Verification items for the finished model (mm, model axes). A direction names the side the tool comes from. Coordinates: 2 decimals unless noted, no trailing zeros. Order: outer loops, then holes, each group sorted by start corner. A loop starts at its lowest first (then second) coordinate and runs counter-clockwise, first axis right, second up. Notation, with made-up numbers: (20, 8) -> (58, 8) arc R25 ccw to (58, 28) -> close; hole circle Ø6 at (27.5, 29). An arc over 180 degrees is marked (long way). Write each question's results on one line, items separated by ' | '. Start each with the question number.
(1) Cross-section at B-B on x = 9.5. Enter the section's corners in (y, z).
(2) Thickness scan on probe 1 along Z at (x, y) = (9.5, 1.35); probe 2 along X at (y, z) = (3.3, 0.25); probe 3 along X at (y, z) = (-0.5, 0.75). Record the ranges inside material, lowest first. Write a range as [from, to].
(3) Set-up check for faces 1 (the flat face through (0, 2, 5)), 2 (the flat face through (6, -0.5, -0.1)): record each of +Z, -Z, +X, -X, +Y, -Y from which the full face is reachable in a straight line by a thin tool's end or side.
(4) Cross-section at C-C on y = 0.3. Enter the section's corners in (x, z).
(5) Draft check along X on faces 3 (the cylindrical face through (12.699, 1.465, -4.715)), 4 (the flat face through (0, 0, 0)), 5 (the flat face through (0, 4, 0)). Enter one of: +X half, -X half, draft (parallel to the pull), parting line (faces both ways), or undercut.
(6) Go/stop test with a flat-tipped pin: pin 1 (1 mm diameter, centred on x = 0.5, z = 2, fed in from -Y). Record where the tip stops, or that it passes through.
(7) Cross-section at D-D on z = -2.25. Enter the section's corners in (x, y).
(8) Cross-section at A-A on z = 0. Enter the section's corners in (x, y), and give its area (3 significant figures).
```python
from build123d import *

# Parameters (mm, degrees)
SKETCH_2_W          = 26
SKETCH_2_H          = 10
EXTRUDE_1_DEPTH     = 4
SKETCH_3_W          = 7
SKETCH_3_H          = 10
EXTRUDE_2_DEPTH     = 1
SKETCH_4_R          = 1.6
CUT_EXTRUDE_1_DEPTH = 6
FILLET_1_R          = 1


with BuildPart() as part:
    # 草图2 → 凸台-拉伸1 (new body)
    with BuildSketch(Plane(origin=(0, 0, 0), x_dir=(1, 0, 0), z_dir=(0, 1, 0))):
        Rectangle(SKETCH_2_W, SKETCH_2_H)
    extrude(amount=EXTRUDE_1_DEPTH)

    # 草图3 → 凸台-拉伸2 (add)
    with BuildSketch(Plane.XZ):
        with Locations((9.5, 0)):
            Rectangle(SKETCH_3_W, SKETCH_3_H)
        with Locations((-9.5, 0)):
            Rectangle(SKETCH_3_W, SKETCH_3_H)
    extrude(amount=EXTRUDE_2_DEPTH)

    # 草图4 → 切除-拉伸1 (cut, through all)
    with BuildSketch(Plane.XZ.offset(1)):
        with Locations((9.5, 0)):
            Circle(SKETCH_4_R)
        with Locations((-9.5, 0)):
            Circle(SKETCH_4_R)
    extrude(amount=-CUT_EXTRUDE_1_DEPTH, mode=Mode.SUBTRACT)

    # 圆角1
    fillet_1_edges = [part.edges().sort_by_distance(p)[0] for p in [
        (13, 1.5, 5),
        (-13, 1.5, 5),
        (-13, 1.5, -5),
        (13, 1.5, -5),
    ]]
    fillet(fillet_1_edges, radius=FILLET_1_R)


solid = part.part
```
Results are:
1) outline: (-1, -5) -> (4, -5) -> (4, -1.6) -> (-1, -1.6) -> close; (-1, 1.6) -> (4, 1.6) -> (4, 5) -> (-1, 5) -> close
2) probe 1: z = [-5, -1.6], [1.6, 5] | probe 2: x = [-13, -11.08], [-7.92, 7.92], [11.08, 13] | probe 3: x = [-13, -10.91], [-8.09, -6], [6, 8.09], [10.91, 13]
3) face 1: +Z, +X, -X, +Y, -Y | face 2: +Z, -Z, -Y
4) outline: (-13, -4) arc R1 ccw to (-12, -5) -> (12, -5) arc R1 ccw to (13, -4) -> (13, 4) arc R1 ccw to (12, 5) -> (-12, 5) arc R1 ccw to (-13, 4) -> close; hole circle Ø3.2 at (-9.5, 0); hole circle Ø3.2 at (9.5, 0)
5) face 3: +X half | face 4: undercut | face 5: draft
6) pin 1: stops at y = 0
7) outline: (-13, -1) -> (-6, -1) -> (-6, 0) -> (6, 0) -> (6, -1) -> (13, -1) -> (13, 4) -> (-13, 4) -> close
8) outline: (-13, -1) -> (-11.1, -1) -> (-11.1, 4) -> (-13, 4) -> close; (-7.9, -1) -> (-6, -1) -> (-6, 0) -> (6, 0) -> (6, -1) -> (7.9, -1) -> (7.9, 4) -> (-7.9, 4) -> close; (11.1, -1) -> (13, -1) -> (13, 4) -> (11.1, 4) -> close | area: 86.0 mm2
